```python
from build123d import *

# Parameters (mm, degrees)
SKETCH3_W           = 20
SKETCH3_H           = 20
BOSS_EXTRUDE1_DEPTH = 25
SKETCH4_R           = 3.75
CUT_EXTRUDE1_DEPTH  = 29.722813233
SKETCH4_3_R         = 6.7
CUT_EXTRUDE2_DEPTH  = 5.5
CUT_EXTRUDE3_START  = -19.5
SKETCH4_4_R         = 6.7
CUT_EXTRUDE3_DEPTH  = 5.5
FILLET1_R           = 1
FILLET2_R           = 1


with BuildPart() as part:
    # Sketch3 → Boss-Extrude1 (new body)
    with BuildSketch(Plane(origin=(0, 0, 0), x_dir=(1, 0, 0), z_dir=(0, 1, 0))):
        Rectangle(SKETCH3_W, SKETCH3_H)
    extrude(amount=BOSS_EXTRUDE1_DEPTH)

    # Sketch4 → Cut-Extrude1 (cut, through all)
    with BuildSketch(Plane(origin=(0, 25, 0), x_dir=(1, 0, 0), z_dir=(0, 1, 0))):
        with Locations(Location((0, 0, 0), (0, 0, 270))):
            Circle(SKETCH4_R)
    extrude(amount=-CUT_EXTRUDE1_DEPTH, mode=Mode.SUBTRACT)

    # Sketch4<3> → Cut-Extrude2 (cut)
    with BuildSketch(Plane(origin=(0, 25, 0), x_dir=(1, 0, 0), z_dir=(0, 1, 0))):
        with Locations(Location((0, 0, 0), (0, 0, 270))):
            Circle(SKETCH4_3_R)
    extrude(amount=-CUT_EXTRUDE2_DEPTH, mode=Mode.SUBTRACT)

    # Sketch4<4> → Cut-Extrude3 (cut)
    with BuildSketch(Plane(origin=(0, 25, 0), x_dir=(1, 0, 0), z_dir=(0, 1, 0)).offset(CUT_EXTRUDE3_START)):
        with Locations(Location((0, 0, 0), (0, 0, 270))):
            Circle(SKETCH4_4_R)
    extrude(amount=-CUT_EXTRUDE3_DEPTH, mode=Mode.SUBTRACT)

    # Fillet1
    fillet1_edges = [part.edges().sort_by_distance(p)[0] for p in [
        (0, 25, -6.7),
        (0, 0, -6.7),
    ]]
    fillet(fillet1_edges, radius=FILLET1_R)

    # Fillet2
    fillet2_edges = [part.edges().sort_by_distance(p)[0] for p in [
        (0, 19.5, -3.75),
        (0, 5.5, -3.75),
    ]]
    fillet(fillet2_edges, radius=FILLET2_R)


solid = part.part
```
Design review of the part built by this model. Coordinates are the model's own, in mm. A direction names the side the tool comes from. Coordinates: 2 decimals unless noted, no trailing zeros. Order: outer loops, then holes, each group sorted by start corner. A loop starts at its lowest first (then second) coordinate and runs counter-clockwise, first axis right, second up. Notation, with made-up numbers: (27.25, -37.75) - (60.25, -37.75) arc R10 cw to (60.25, -32.75) - close; hole circle Ø8 at (7.25, 23.5). An arc over 180 degrees is marked (long way). Answer in a Markdown table with one row per item.
(1) Consider section B-B on x = 0. State the section outline as (y, z) points, plus the area to 3 significant figures.
Checked values:
| item | result |
|---|---|
| outline | (0, -10) - (25, -10) - (25, -7.7) arc R1 ccw to (24, -6.7) - (19.5, -6.7) - (19.5, -4.75) arc R1 ccw to (18.5, -3.75) - (6.5, -3.75) arc R1 ccw to (5.5, -4.75) - (5.5, -6.7) - (1, -6.7) arc R1 ccw to (0, -7.7) - close; (0, 7.7) arc R1 ccw to (1, 6.7) - (5.5, 6.7) - (5.5, 4.75) arc R1 ccw to (6.5, 3.75) - (18.5, 3.75) arc R1 ccw to (19.5, 4.75) - (19.5, 6.7) - (24, 6.7) arc R1 ccw to (25, 7.7) - (25, 10) - (0, 10) - close |
| area | 246 mm^2 |
(2) Consider section A-A on z = 0. State the section outline as (x, y) points, plus the area to 3 significant figures.
Checked values:
| item | result |
|---|---|
| outline | (-10, 0) - (-7.7, 0) arc R1 ccw to (-6.7, 1) - (-6.7, 5.5) - (-4.75, 5.5) arc R1 ccw to (-3.75, 6.5) - (-3.75, 18.5) arc R1 ccw to (-4.75, 19.5) - (-6.7, 19.5) - (-6.7, 24) arc R1 ccw to (-7.7, 25) - (-10, 25) - close; (3.75, 6.5) arc R1 ccw to (4.75, 5.5) - (6.7, 5.5) - (6.7, 1) arc R1 ccw to (7.7, 0) - (10, 0) - (10, 25) - (7.7, 25) arc R1 ccw to (6.7, 24) - (6.7, 19.5) - (4.75, 19.5) arc R1 ccw to (3.75, 18.5) - close |
| area | 246 mm^2 |
(3) Consider section D-D on y = 10. State the section outline as (x, z) points, plus the area to 3 significant figures.
Checked values:
| item | result |
|---|---|
| outline | (-10, -10) - (10, -10) - (10, 10) - (-10, 10) - close; hole circle Ø7.5 at (0, 0) |
| area | 356 mm^2 |
(4) Clearance check with flat-ended pins moving along their axes: pin 1 (10 mm diameter, centred on x = 0, z = 0, fed in from -Y); pin 2 (10.5 mm diameter, centred on x = 0, z = 0, fed in from +Y). State where each tip first meets the part, or that it passes through.
Checked values:
| item | result |
|---|---|
| pin 1 | y = 5.5 |
| pin 2 | y = 19.5 |
(5) For faces 1 (the flat face through (5, 5.5, 1)), 2 (the flat face through (5, 19.5, 1)), 3 (the flat face through (0, 12, -10)), list the 3-axis set-ups (+Z, -Z, +X, -X, +Y, -Y) from which the entire face can be reached by the end or side of a thin tool; tool diameter is ignored.
Checked values:
| item | result |
|---|---|
| face 1 | -Y |
| face 2 | +Y |
| face 3 | -Z, +X, -X, +Y, -Y |
(6) The part is to be moulded in two halves that separate along Z. For faces 4 (the flat face through (-10, 12, 0)), 5 (the cylindrical face through (-4.1, 21.8, -5.3)), 6 (the flat face through (0, 12, 10)), say which applies: released by +Z, released by -Z, zero draft, split by the parting line, or undercut.
Checked values:
| item | result |
|---|---|
| face 4 | zero draft |
| face 5 | undercut |
| face 6 | released by +Z |
(7) Wall thickness on line 1 along X through (y, z) = (12, 0); line 2 along X through (y, z) = (21.5, 0); line 3 along Y through (x, z) = (4.75, 1): over which ranges is each line inside the solid? List them lowest first. Write a range as from..to.
Checked values:
| item | result |
|---|---|
| line 1 | -10..-3.75, 3.75..10 |
| line 2 | -10..-6.7, 6.7..10 |
| line 3 | 5.5..19.5 |
(8) Consider section C-C on y = 5. State the section outline as (x, z) points.
Checked values:
| item | result |
|---|---|
| outline | (-10, -10) - (10, -10) - (10, 10) - (-10, 10) - close; hole circle Ø13.4 at (0, 0) |
